Can you work these out from the drawing? Everything is in mm from the part's minimum corner. A direction names the side the tool comes from. Coordinates: 2 decimals unless noted, no trailing zeros. Order: outer loops, then holes, each group sorted by start corner. A loop starts at its lowest first (then second) coordinate and runs counter-clockwise, first axis right, second up. Notation, with made-up numbers: (75, 42.5) -> (124, 42.5) arc R11 cw to (124, 52.5) -> close; hole circle Ø9 at (17, 44). An arc over 180 degrees is marked (long way). Answer in a Markdown table with one row per item.
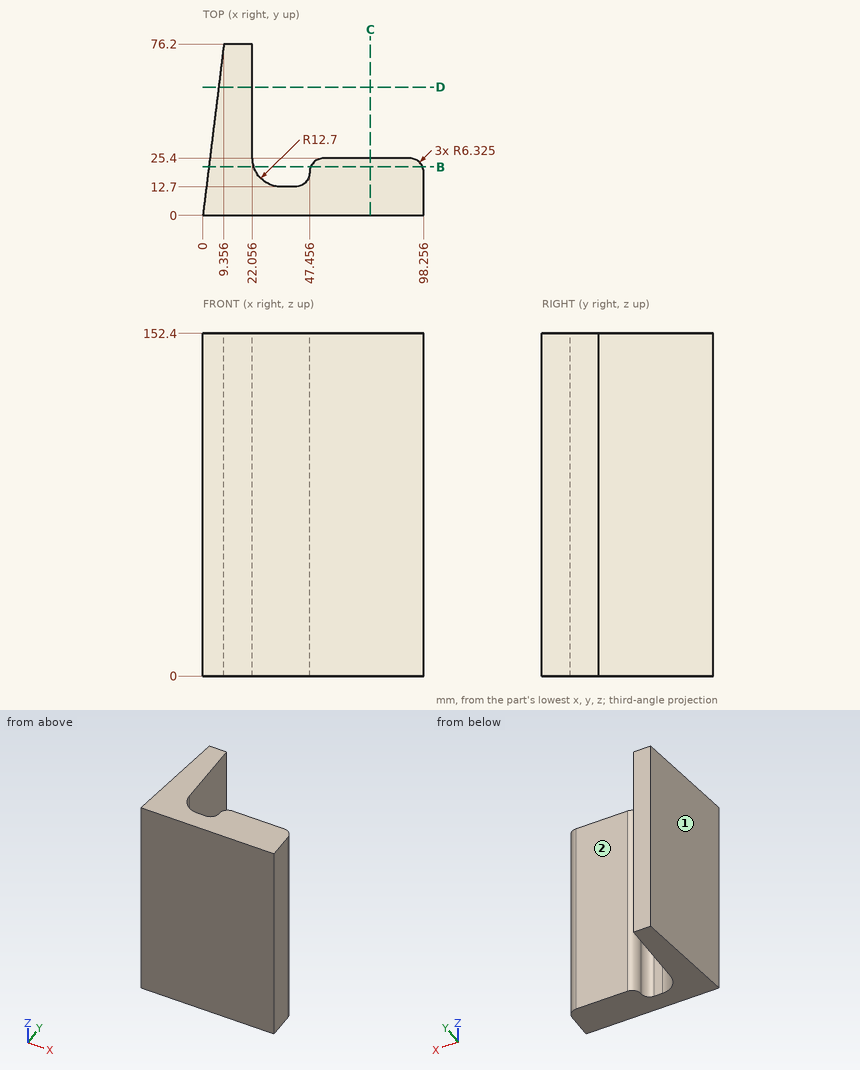
(1) I need wall thicknesses on line 1 (Y direction, x = 64, z = 121); line 2 (Y direction, x = 38.5, z = 22); line 3 (X direction, y = 21, z = 82) (1 decimal). Which ranges of each line are inside material? Lowest first, please. Write a range as [from, to].
Response values:
| item | result |
|---|---|
| line 1 | [0, 25.4] |
| line 2 | [0, 12.7] |
| line 3 | [2.6, 22.8], [47.8, 98] |
(2) Will these pins go through, and if not, where does the flat tip stop? pin 1 Ø5 at (x, z) = (36.5, 106.5) entering from +Y; pin 2 Ø11.5 at (x, z) = (74.5, 75) entering from +Y.
Response values:
| item | result |
|---|---|
| pin 1 | y = 12.72 |
| pin 2 | y = 25.4 |
(3) Suppose I cut it at C-C (x = 74.5). Please give me the cut outline in (y, z).
Response values:
| item | result |
|---|---|
| outline | (0, 0) -> (25.4, 0) -> (25.4, 152.4) -> (0, 152.4) -> close |
(4) Suppose I cut it at D-D (y = 57). Please give me the cut outline in (x, z).
Response values:
| item | result |
|---|---|
| outline | (7, 0) -> (22.06, 0) -> (22.06, 152.4) -> (7, 152.4) -> close |
(5) Suppose I cut it at B-B (y = 21.5). Please give me the cut outline in (x, z), and give its area (3 significant figures).
Response values:
| item | result |
|---|---|
| outline | (2.64, 0) -> (22.67, 0) -> (22.67, 152.4) -> (2.64, 152.4) -> close; (47.94, 0) -> (97.77, 0) -> (97.77, 152.4) -> (47.94, 152.4) -> close |
| area | 10,600 mm2 |
(6) On a 3-axis mill with a long thin cutter (end or side, diameter ignored), from which of +Z, -Z, +X, -X, +Y, -Y can I reach the whole of each face in a straight line? I mean the marked faces 1 and 2. Say none if no direction works.
Response values:
| item | result |
|---|---|
| face 1 | +Z, -Z, -X, +Y |
| face 2 | +Z, -Z, +X, +Y |
